from build123d import *

# Parameters (mm, degrees)
F1_DEPTH = 15
F2_W     = 10
F2_H     = 10
F3_DEPTH = 25


with BuildPart() as f1:
    # F0 (on Front) → F1 (new body)
    with BuildSketch(Plane.XZ):
        Polygon((12.5, 0), (0, 0), (0, -20), (5, -20), (5, -17.5), (20, -17.5), (20, -20), (30, -20), (30, -10), align=None)
    extrude(amount=-F1_DEPTH)

    # F2 (on face) → F3 (cut)
    with BuildSketch(Plane.XY):
        with Locations((25, 7.5)):
            Rectangle(F2_W, F2_H)
    extrude(amount=-F3_DEPTH, mode=Mode.SUBTRACT)


solid = f1.part
Can you work these out from the model? Positions are in its coordinate system, mm. A direction names the side the tool comes from. Coordinates: 2 decimals unless noted, no trailing zeros. Write each loop counter-clockwise with the first axis right and the second up, starting at its lowest first coordinate (ties: lowest second). Pieces come first, ordered by that corner, then holes. Notation, with made-up numbers: (29.5, 35.5) - (43.5, 35.5) arc R26 ccw to (43.5, 49.5) - close; hole circle Ø4 at (-26, -15). An arc over 180 degrees is marked (long way). Return JSON: item names as keys, results as strings. Group by question number.
Item 1: Please list where these lines run through material, in increasing order: probe 1 along Y at (x, z) = (22, -17.75); probe 2 along X at (y, z) = (4, -4.5); probe 3 along X at (y, z) = (11.5, -19).
Item 2: If we section it at A-A (z = -18): Write out the boundary of the cut face in (x, y), then the cut area to 3 significant figures.
Item 3: If we section it at C-C (y = 11.5): Write out the boundary of the cut face in (x, z).
Item 4: We'd pull the mould along X, two halves only. Please class faces 4 (the face through (19.43, 7.4, -3.96)), 5 (the face through (12, 7, -17.5)), 6 (the face through (25, 2.5, -14)), 7 (the face through (20, 14, -19)): pulls with the +X half, pulls with the -X half, needs draft (parallel to the pull), parting line crosses it, or undercut.
Item 5: I'm going to push flat-ended pins straight in: pin 1 Ø5 at (y, z) = (6.5, -12) entering from +X; pin 2 Ø1.5 at (x, y) = (10.5, 2.5) entering from -Z; pin 3 Ø2 at (y, z) = (8, -19) entering from +X. Where does each tip first touch, or does it pass through?
Item 6: If we section it at D-D (z = -12.5): Write out the boundary of the cut face in (x, y), then the cut area to 3 significant figures.
Item 7: If we section it at B-B (x = 21.25): Write out the boundary of the cut face in (y, z).
Item 8: Which directions (+Z, -Z, +X, -X, +Y, -Y) give clear straight access to the entire face, cutting with the end or side of a thin tool? Please do faces 1 (the face through (6, 7, 0)), 2 (the face through (25, 12.5, -14)), 3 (the face through (5, 7, -19)).
Return value:
{
 "1": {"probe 1": "y = 0 to 2.5, 12.5 to 15", "probe 2": "x = 0 to 20", "probe 3": "x = 0 to 5"},
 "2": {"outline": "(0, 0) - (5, 0) - (5, 15) - (0, 15) - close; (20, 0) - (30, 0) - (30, 2.5) - (20, 2.5) - close; (20, 12.5) - (30, 12.5) - (30, 15) - (20, 15) - close", "area": "125 mm^2"},
 "3": {"outline": "(0, -20) - (5, -20) - (5, -17.5) - (20, -17.5) - (20, -4.29) - (12.5, 0) - (0, 0) - close"},
 "4": {"face 4": "pulls with the +X half", "face 5": "undercut", "face 6": "needs draft", "face 7": "undercut"},
 "5": {"pin 1": "stops at x = 20", "pin 2": "stops at z = -17.5", "pin 3": "stops at x = 5"},
 "6": {"outline": "(0, 0) - (30, 0) - (30, 2.5) - (20, 2.5) - (20, 12.5) - (30, 12.5) - (30, 15) - (0, 15) - close", "area": "350 mm^2"},
 "7": {"outline": "(0, -20) - (2.5, -20) - (2.5, -5) - (0, -5) - close; (12.5, -20) - (15, -20) - (15, -5) - (12.5, -5) - close"},
 "8": {"face 1": "+Z, +X, -X, +Y, -Y", "face 2": "+Z, -Z, +X", "face 3": "-Z, +Y, -Y"}
}
